from build123d import *

# Parameters (mm, degrees)
SKETCH1_R           = 2.5
SKETCH1_R_2         = 4
BOSS_EXTRUDE1_DEPTH = 3


with BuildPart() as part:
    # Sketch1 → Boss-Extrude1 (new body)
    with BuildSketch(Plane(origin=(0, 0, 0), x_dir=(1, 0, 0), z_dir=(0, 1, 0))):
        with BuildLine():
            Line((-56, 14.25), (-63.418747228, 14.25))
            ThreePointArc((-63.418747228, 14.25), (-45.961940777, 45.961940777), (-14.25, 63.418747228))
            Line((-14.25, 63.418747228), (-14.25, 56))
            ThreePointArc((-14.25, 56), (0, 41.75), (14.25, 56))
            Line((14.25, 56), (14.25, 63.418747228))
            ThreePointArc((14.25, 63.418747228), (45.961940777, 45.961940777), (63.418747228, 14.25))
            Line((63.418747228, 14.25), (56, 14.25))
            ThreePointArc((56, 14.25), (41.75, 0), (56, -14.25))
            Line((56, -14.25), (63.418747228, -14.25))
            ThreePointArc((63.418747228, -14.25), (45.961940777, -45.961940777), (14.25, -63.418747228))
            Line((14.25, -63.418747228), (14.25, -56))
            ThreePointArc((14.25, -56), (0, -41.75), (-14.25, -56))
            Line((-14.25, -56), (-14.25, -63.418747228))
            ThreePointArc((-14.25, -63.418747228), (-45.961940777, -45.961940777), (-63.418747228, -14.25))
            Line((-63.418747228, -14.25), (-56, -14.25))
            ThreePointArc((-56, -14.25), (-41.75, 0), (-56, 14.25))
        make_face()
        with Locations(Location((-31.819805153, 31.819805153, 0), (0, 0, 270))):
            Circle(SKETCH1_R, mode=Mode.SUBTRACT)
        with Locations(Location((31.819805153, 31.819805153, 0), (0, 0, 270))):
            Circle(SKETCH1_R, mode=Mode.SUBTRACT)
        with Locations(Location((31.819805153, -31.819805153, 0), (0, 0, 270))):
            Circle(SKETCH1_R, mode=Mode.SUBTRACT)
        with Locations(Location((-31.819805153, -31.819805153, 0), (0, 0, 270))):
            Circle(SKETCH1_R, mode=Mode.SUBTRACT)
        with Locations(Location((0, 0, 0), (0, 0, 270))):
            Circle(SKETCH1_R_2, mode=Mode.SUBTRACT)
    extrude(amount=BOSS_EXTRUDE1_DEPTH)


solid = part.part
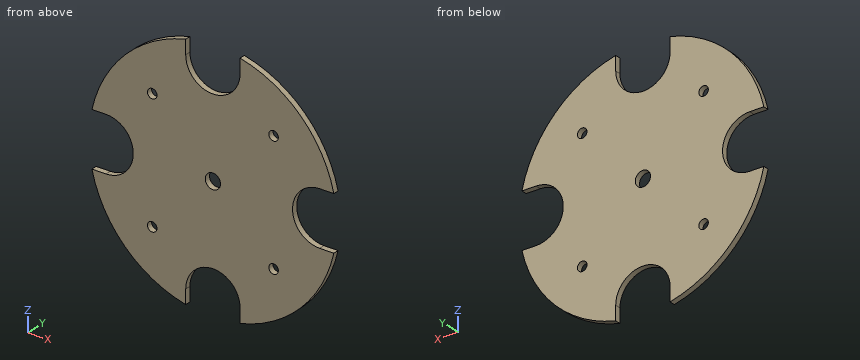
Input: part model. Units: mm. Frame: model coordinates. Round coordinates to 2 decimals unless told otherwise and drop trailing zeros. Loops run counter-clockwise (first coordinate to the right, second up) from the corner with the lowest first, then second, coordinate; pieces in that order, holes last. Notation, with made-up numbers: M 73,20 L 90,20 A18 ccw 90,37 Z; hole C 63,11 d10. An arc over 180 degrees is marked long. Answer as CSV lines item,"result". Start each with the question number.
(1) Line query: line 1 (Z direction, x = -31, y = 2.6); line 2 (X direction, y = 2.35, z = 0); line 3 (Z direction, x = -49, y = 2.85). Output: solid intervals per line, ascending. Write a range as [from, to].
(2) First-contact query: pin 1 (1.5 mm diameter, centred on y = 0.5, z = -29, fed in from +X); pin 2 (0.9 mm diameter, centred on x = -59.5, y = 1.5, fed in from -Z); pin 3 (0.9 mm diameter, centred on x = -59.5, y = 1, fed in from +Z); pin 4 (6 mm diameter, centred on x = -31.82, z = -31.82, fed in from -Y). Flat tips, straight axial feed; report the tip coordinate or a pass-through.
(3) Section A-A, the plane x = 0. Output: boundary loops of the cut face in (y, z).
(4) Section D-D, the plane z = 20. Output: boundary loops of the cut face in (x, y), plus the area to 3 significant figures.
(5) Section C-C, the plane y = 2.55. Output: boundary loops of the cut face in (x, z), plus the area to 3 significant figures.
(6) Section B-B, the plane z = 0. Output: boundary loops of the cut face in (x, y), plus the area to 4 significant figures.
Values found:
1,line 1,"z = [-57.13, -34.18], [-29.46, 29.46], [34.18, 57.13]"
1,line 2,"x = [-41.75, -4], [4, 41.75]"
1,line 3,"z = [-42.71, -12.41], [12.41, 42.71]"
2,pin 1,"stops at x = 58.54"
2,pin 2,"stops at z = -27.17"
2,pin 3,"stops at z = 27.17"
2,pin 4,"stops at y = 0"
3,outline,"M 0,-41.75 L 3,-41.75 L 3,-4 L 0,-4 Z; M 0,4 L 3,4 L 3,41.75 L 0,41.75 Z"
4,outline,"M -61.85,0 L 61.85,0 L 61.85,3 L -61.85,3 Z"
4,area,"371 mm²"
5,outline,"M -63.42,-14.25 A65 ccw -14.25,-63.42 L -14.25,-56 A14.25 cw 14.25,-56 L 14.25,-63.42 A65 ccw 63.42,-14.25 L 56,-14.25 A14.25 cw 56,14.25 L 63.42,14.25 A65 ccw 14.25,63.42 L 14.25,56 A14.25 cw -14.25,56 L -14.25,63.42 A65 ccw -63.42,14.25 L -56,14.25 A14.25 cw -56,-14.25 Z; hole C -31.82,-31.82 d5; hole C -31.82,31.82 d5; hole C 0,0 d8; hole C 31.82,-31.82 d5; hole C 31.82,31.82 d5"
5,area,"10,900 mm²"
6,outline,"M -41.75,0 L -4,0 L -4,3 L -41.75,3 Z; M 4,0 L 41.75,0 L 41.75,3 L 4,3 Z"
6,area,"226.5 mm²"
